The model under review builds one solid part; all positions refer to its coordinate system, in mm. Face numbers are marked on the shaded views. A direction names the side the tool comes from. Give positions to 0.01 mm unless a question says otherwise; leave off trailing zeros. Write each loop counter-clockwise with the first axis right and the second up, starting at its lowest first coordinate (ties: lowest second). Pieces come first, ordered by that corner, then holes.
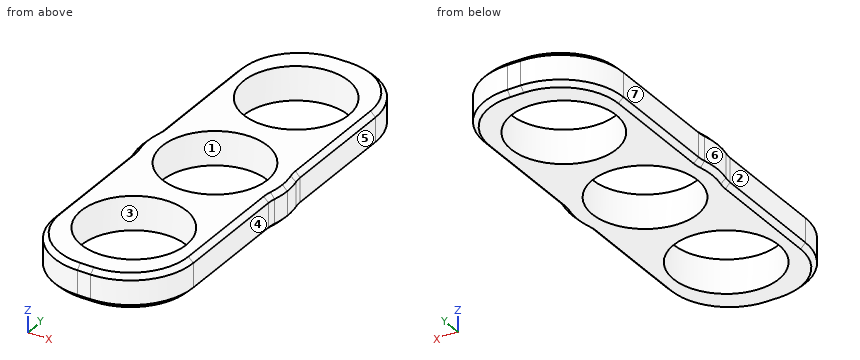
from build123d import *

# Parameters (mm, degrees)
F0_R     = 10.925
F1_DEPTH = 3.5
F2_R     = 13
F3_R     = 7
F4_SIZE  = 1


with BuildPart() as f1:
    # F0 (on Top) → F1 (new body, symmetric)
    with BuildSketch(Plane.XY):
        with BuildLine():
            ThreePointArc((-14.387438, 4.242832), (0, 15), (14.387438, 4.242832))
            Line((14.387438, 4.242832), (14.387438, 42.63803))
            Line((14.387438, 42.63803), (-14.387438, 42.63803))
            Line((-14.387438, 42.63803), (-14.387438, 4.242832))
        make_face()
        with Locations((0, 26.42202)):
            Circle(F0_R, mode=Mode.SUBTRACT)
        with BuildLine():
            ThreePointArc((14.387438, -4.242832), (14.84607, -2.143412), (15, 0))
            ThreePointArc((15, 0), (14.84607, 2.143412), (14.387438, 4.242832))
            ThreePointArc((14.387438, 4.242832), (0, 15), (-14.387438, 4.242832))
            ThreePointArc((-14.387438, 4.242832), (-15, 0), (-14.387438, -4.242832))
            ThreePointArc((-14.387438, -4.242832), (0, -15), (14.387438, -4.242832))
        make_face()
        Circle(F0_R, mode=Mode.SUBTRACT)
        with BuildLine():
            Line((14.387438, -42.63803), (14.387438, -4.242832))
            ThreePointArc((14.387438, -4.242832), (0, -15), (-14.387438, -4.242832))
            Line((-14.387438, -4.242832), (-14.387438, -42.63803))
            Line((-14.387438, -42.63803), (14.387438, -42.63803))
        make_face()
        with Locations((0, -26.42202)):
            Circle(F0_R, mode=Mode.SUBTRACT)
    extrude(amount=F1_DEPTH, both=True)

    # F2
    f2_edges = [f1.edges().sort_by_distance(p)[0] for p in [
        (-14.387438, 42.63803, 0),
        (14.387438, 42.63803, 0),
        (14.387438, -42.63803, 0),
        (-14.387438, -42.63803, 0),
    ]]
    fillet(f2_edges, radius=F2_R)

    # F3
    f3_edges = [f1.edges().sort_by_distance(p)[0] for p in [
        (14.387438, -4.242832, -1.75),
        (14.387438, 4.242832, -1.75),
        (-14.387438, 4.242832, 0),
        (-14.387438, -4.242832, 0),
    ]]
    fillet(f3_edges, radius=F3_R)

    # F4
    f4_edges = [f1.edges().sort_by_distance(p)[0] for p in [
        (14.387438, -17.396683, 3.5),
        (14.387438, -17.396683, -3.5),
    ]]
    chamfer(f4_edges, length=F4_SIZE)


solid = f1.part
1) Tool access review of the marked faces 5, 6 and 7: name each direction out of +Z, -Z, +X, -X, +Y, -Y from which nothing blocks a thin tool from reaching the whole face with its end or side.
2) Insertion check: pin 1 (1.5 mm diameter, centred on y = -23.5, z = -0.5, fed in from -X); pin 2 (1.5 mm diameter, centred on x = -3.5, z = -1, fed in from -Y); pin 3 (1.5 mm diameter, centred on y = -11.5, z = 0.5, fed in from +X). Each pin has a flat end and moves straight along its axis. Give the tip position at first contact, or say it passes through.
3) Consider section D-D, the plane x = 5.5. State how many separate pieces and enclosed holes the cut face has, then the cut area to 3 significant figures.
4) To check wall thickness, follow probe 1 along Y at (x, z) = (0, 1.75) (3 decimals); probe 2 along X at (y, z) = (-26, -2); probe 3 along Y at (x, z) = (1.5, 0.5). State the ranges of each line that lie inside material, in increasing order.
5) Consider section A-A, the plane x = 0. Give the boundary of the cut face in (y, z) (3 decimals).
6) Consider section C-C, the plane y = 27.5. Give the boundary of the cut face in (x, z), then the cut area to 3 significant figures.
7) Consider section B-B, the plane z = -1.5. Give the boundary of the cut face in (x, y) (3 decimals).
8) The part is to be moulded in two halves that separate along X. For the marked faces 1, 2, 3 and 4, say which applies: +X half, -X half, draft (parallel to the pull), parting line (faces both ways), or undercut.
Answer block:
1. face 5: +Z, -Z, +X, +Y
1. face 6: +Z, -Z, -X
1. face 7: +Z, -Z, -X, +Y
2. pin 1: stops at x = -14.39
2. pin 2: stops at y = -42.57
2. pin 3: stops at x = 14.39
3. separate pieces: 4
3. enclosed holes: 0
3. area: 189 mm2
4. probe 1: y = -42.638 to -37.347, -15.497 to -10.925, 10.925 to 15.497, 37.347 to 42.638
4. probe 2: x = -14.39 to -10.92, 10.92 to 14.39
4. probe 3: y = -42.64 to -37.24, -15.6 to -10.82, 10.82 to 15.6, 37.24 to 42.64
5. outline: (-42.638, -2.5) - (-41.638, -3.5) - (-37.347, -3.5) - (-37.347, 3.5) - (-41.638, 3.5) - (-42.638, 2.5) - close; (-15.497, -3.5) - (-10.925, -3.5) - (-10.925, 3.5) - (-15.497, 3.5) - close; (10.925, -3.5) - (15.497, -3.5) - (15.497, 3.5) - (10.925, 3.5) - close; (37.347, -3.5) - (41.638, -3.5) - (42.638, -2.5) - (42.638, 2.5) - (41.638, 3.5) - (37.347, 3.5) - close
6. outline: (-14.39, -2.5) - (-13.39, -3.5) - (-10.87, -3.5) - (-10.87, 3.5) - (-13.39, 3.5) - (-14.39, 2.5) - close; (10.87, -3.5) - (13.39, -3.5) - (14.39, -2.5) - (14.39, 2.5) - (13.39, 3.5) - (10.87, 3.5) - close
6. area: 47.2 mm2
7. outline: (-14.582, -3.515) arc R7 cw to (-14.387, -5.155) - (-14.387, -29.638) arc R13 ccw to (-1.387, -42.638) - (1.387, -42.638) arc R13 ccw to (14.387, -29.638) - (14.387, -5.155) arc R7 cw to (14.582, -3.515) arc R15 ccw to (15, 0) arc R15 ccw to (14.582, 3.515) arc R7 cw to (14.387, 5.155) - (14.387, 29.638) arc R13 ccw to (1.387, 42.638) - (-1.387, 42.638) arc R13 ccw to (-14.387, 29.638) - (-14.387, 5.155) arc R7 cw to (-14.582, 3.515) arc R15 ccw to start; hole circle Ø21.85 at (0, -26.422); hole circle Ø21.85 at (0, 0); hole circle Ø21.85 at (0, 26.422)
8. face 1: undercut
8. face 2: -X half
8. face 3: undercut
8. face 4: +X half
